Part model, mm, in its own coordinate system. Face numbers are marked on the shaded views. A direction names the side the tool comes from. Coordinates: 2 decimals unless noted, no trailing zeros. Loops run counter-clockwise (first coordinate to the right, second up) from the corner with the lowest first, then second, coordinate; pieces in that order, holes last. Notation, with made-up numbers: (26.5, 2) - (31.5, 2) arc R20 ccw to (31.5, 13) - close; hole circle Ø2 at (-35.75, 54). An arc over 180 degrees is marked (long way). Use a Markdown table: item, result. Add a question column.
1) Band-saw the part on A-A (y = -8). Give the cut face in (x, z).
2) Band-saw the part on D-D (y = 7). Give the cut face in (x, z), plus the area to 4 significant figures.
3) Drop flat-ended pins along their axis: P1, Ø5, axis at x = -8, y = -8, coming from the -Z side; P2, Ø1.5, axis at x = 11, y = -13, coming from the +Z side. Give the stop position or say it passes through.
4) Probe probe 1 along Y at (x, z) = (-8, 7); probe 2 along Z at (x, y) = (7, 10); probe 3 along Y at (x, z) = (-17, 26). List the from-to ranges inside material, lowest first. Write a range as [from, to].
5) Band-saw the part on C-C (z = 23.5). Give the cut face in (x, y).
6) Tool access for the marked faces 1 and 2: list every direction of +Z, -Z, +X, -X, +Y, -Y with a clear straight run to the whole face (end or side of a thin tool).
7) Pull direction Y, two halves, no side cores. Call the marked faces 3, 4 and 5: +Y half, -Y half, draft (parallel to the pull), parting line (faces both ways), or undercut.
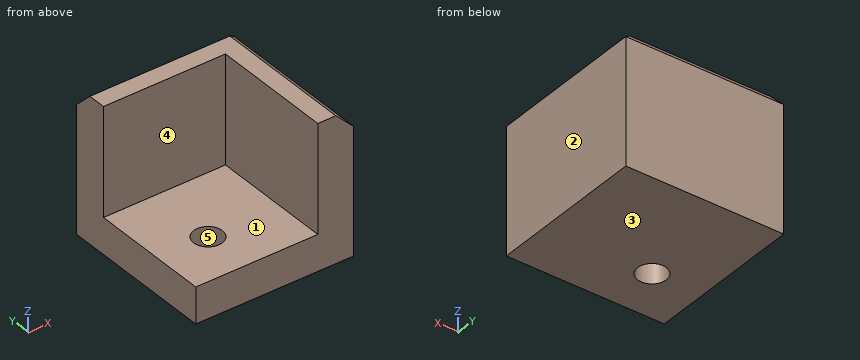
Solid Edge part; units mm, degrees
sketch "Sketch1" plane through (0, 0, 0) normal (0, 0, 1) x (1, 0, 0)
  line L0 (-22, -22) -> (22, -22)
  line L1 (22, -22) -> (22, 22)
  line L2 (22, 22) -> (-22, 22)
  line L3 (-22, 22) -> (-22, -22)
  dimension "D1" = 22
extrude "Protrusion1" add sketch "Sketch1" along normal blind 40
sketch "Sketch2" plane through (0, 0, 40) normal (0, 0, 1) x (1, 0, 0)
  line L0 (-22, 12) -> (12, 12)
  line L1 (12, 12) -> (12, -22)
  line L2 (12, -22) -> (-22, -22)
  line L3 (-22, -22) -> (-22, 12)
  dimension "D1" = 22
extrude "ExtrudedCutout_1" cut sketch "Sketch2" against normal blind 30
chamfer "Chamfer_1" distance 5 angle 45 2 edges at (22, 0, 40) (0, 22, 40)
sketch "Sketch3" plane through (-5, -5, 10) normal (0, 0, 1) x (1, 0, 0)
  circle A0 centre (-3, -3) radius 4
extrude "Cutout1" cut sketch "Sketch3" against normal through all
properties material "Polyethylene, low density"
Answer block:
| question | item | result |
|---|---|---|
| 1 | outline | (-22, 0) - (-12, 0) - (-12, 10) - (-22, 10) - close; (-4, 0) - (22, 0) - (22, 35) - (17, 40) - (12, 40) - (12, 10) - (-4, 10) - close |
| 2 | outline | (-22, 0) - (22, 0) - (22, 35) - (17, 40) - (12, 40) - (12, 10) - (-22, 10) - close |
| 2 | area | 727.5 mm2 |
| 3 | P1 | through |
| 3 | P2 | z = 10 |
| 4 | probe 1 | [-22, -12], [-4, 22] |
| 4 | probe 2 | [0, 10] |
| 4 | probe 3 | [12, 22] |
| 5 | outline | (-22, 12) - (12, 12) - (12, -22) - (22, -22) - (22, 22) - (-22, 22) - close |
| 6 | face 1 | +Z, -X, -Y |
| 6 | face 2 | +Z, -Z, +X, +Y, -Y |
| 7 | face 3 | draft |
| 7 | face 4 | -Y half |
| 7 | face 5 | undercut |
